from build123d import *

# Parameters (mm, degrees)
F1_DEPTH = 8.382


with BuildPart() as f1:
    # F0 (on Front) → F1 (new body)
    with BuildSketch(Plane.XZ):
        Polygon((-12.636772, 1.991665), (-17.343119, 0.441339), (-24.312051, -1.854309), (-12.636772, -20.397399), (-6.730455, -14.300559), (-4.054186, -11.53796), align=None)
        Polygon((4.395189, 12.306461), (7.302871, 15.307937), (4.944825, 19.435907), (-19.505887, 5.468773), (-18.405734, 2.129021), (-17.343119, 0.441339), (-12.636772, 1.991665), (-4.054186, -11.53796), (-6.730455, -14.300559), (-6.730455, -15.967679), (-4.054186, -19.161193), (18.955158, -5.288215), (16.973184, -2.000967), (15.571872, -0.643444), (12.499417, -1.716953), align=None)
        Polygon((12.499417, 20.672111), (8.241373, 16.276713), (7.302871, 15.307937), (4.395189, 12.306461), (12.499417, -1.716953), (15.571872, -0.643444), (23.899982, 2.266378), align=None)
    extrude(amount=F1_DEPTH)


solid = f1.part
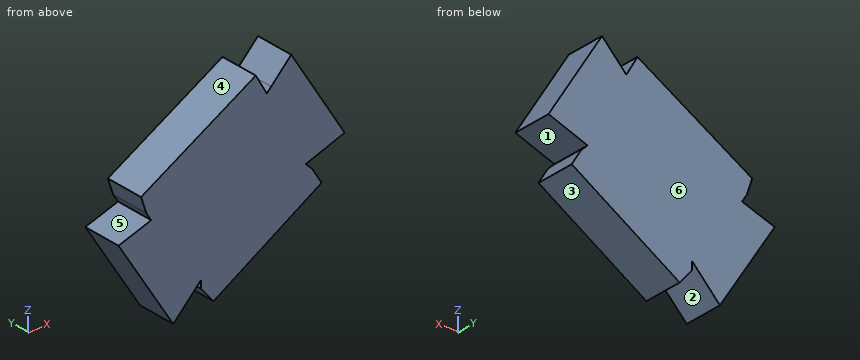
Read the model definition and answer for the solid it produces. Units are mm, in the model's axes. Face numbers are marked on the shaded views. A direction names the side the tool comes from. Coordinates: 2 decimals unless noted, no trailing zeros. Loops run counter-clockwise (first coordinate to the right, second up) from the corner with the lowest first, then second, coordinate; pieces in that order, holes last. Notation, with made-up numbers: (-34, 14) -> (-10, 14) arc R32 ccw to (-10, 45) -> close; hole circle Ø9 at (42.25, 48). An arc over 180 degrees is marked (long way). Answer in a Markdown table with one row per item.
Item 1: Straight lines are drawn through the part: line 1 along X through (y, z) = (-3.5, -15); line 2 along Z through (x, y) = (16, -1.25); line 3 along X through (y, z) = (-4, -7). For each, find the intervals that lie inside material, in ascending order. Write a range as [from, to].
Returned:
| item | result |
|---|---|
| line 1 | x = [-16.04, -7.41], [-6.73, 2.85] |
| line 2 | z = [-7.07, -1.06], [-0.49, 15.02] |
| line 3 | x = [-21.07, 16.12] |
Item 2: For the marked faces 1, 2 and 3, determine the directions among +Z, -Z, +X, -X, +Y, -Y from which every point of the face is accessible in a straight line to the end or side of a thin tool.
Returned:
| item | result |
|---|---|
| face 1 | +X, +Y, -Y |
| face 2 | -Z, +Y, -Y |
| face 3 | -Z, +X, +Y, -Y |
Item 3: A cutting plane is placed at D-D on z = -7.5. Determine the outline of the cut face in (x, y), plus the area to 3 significant figures.
Returned:
| item | result |
|---|---|
| outline | (-20.76, -8.38) -> (15.29, -8.38) -> (15.29, 0) -> (-20.76, 0) -> close |
| area | 302 mm^2 |
Item 4: Each of these flat-tipped pins is pushed along its axis until it touches: P1, Ø1.5, axis at x = -11, z = 12.5, coming from the +Y side; P2, Ø3, axis at x = -16, y = -7, coming from the -Z side; P3, Ø0.5, axis at y = -4, z = -15, coming from the -X side; P4, Ø6, axis at x = 5.5, z = -0.5, coming from the +Y side. Where does it stop, or does it pass through?
Returned:
| item | result |
|---|---|
| P1 | passes through |
| P2 | stops at z = -17.44 |
| P3 | stops at x = -16.19 |
| P4 | stops at y = 0 |
Item 5: A cutting plane is placed at C-C on y = -4.75. Determine the outline of the cut face in (x, z).
Returned:
| item | result |
|---|---|
| outline | (-24.31, -1.85) -> (-12.64, -20.4) -> (-6.73, -14.3) -> (-6.73, -15.97) -> (-4.05, -19.16) -> (18.96, -5.29) -> (16.97, -2) -> (15.57, -0.64) -> (23.9, 2.27) -> (12.5, 20.67) -> (8.24, 16.28) -> (7.3, 15.31) -> (4.94, 19.44) -> (-19.51, 5.47) -> (-18.41, 2.13) -> (-17.34, 0.44) -> close |
Item 6: A cutting plane is placed at A-A on x = 18. Determine the outline of the cut face in (y, z).
Returned:
| item | result |
|---|---|
| outline | (-8.38, -5.86) -> (0, -5.86) -> (0, -3.7) -> (-8.38, -3.7) -> close; (-8.38, 0.2) -> (0, 0.2) -> (0, 11.79) -> (-8.38, 11.79) -> close |
Item 7: For a pull along Z with two mould halves and no side action, classify the marked faces 4, 5 and 6 as released by +Z, released by -Z, zero draft, split by the parting line, or undercut.
Returned:
| item | result |
|---|---|
| face 4 | released by +Z |
| face 5 | undercut |
| face 6 | zero draft |
Item 8: A cutting plane is placed at B-B on z = -17. Determine the outline of the cut face in (x, y).
Returned:
| item | result |
|---|---|
| outline | (-14.78, -8.38) -> (-9.35, -8.38) -> (-9.35, 0) -> (-14.78, 0) -> close; (-5.87, -8.38) -> (-0.47, -8.38) -> (-0.47, 0) -> (-5.87, 0) -> close |
